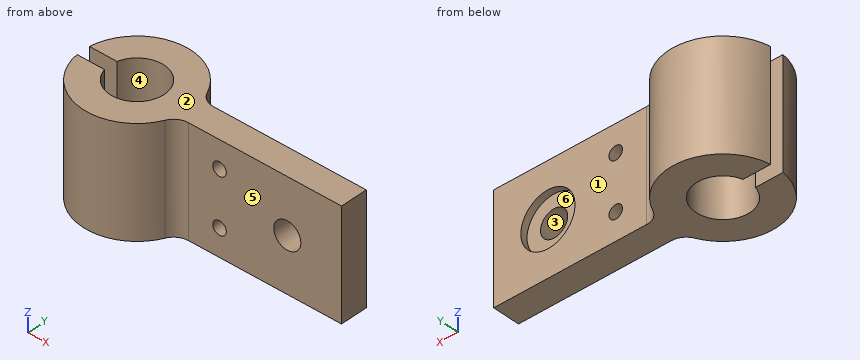
Autodesk Inventor part; units mm, degrees
ref_plane "YZ Plane" through (0, 0, 0) normal (1, 0, 0) x (0, 1, 0)
ref_plane "XZ Plane" through (0, 0, 0) normal (0, 1, 0) x (-1, 0, 0)
ref_plane "XY Plane" through (0, 0, 0) normal (0, 0, 1) x (1, 0, 0)
sketch "Sketch1" plane through (0, 0, 0) normal (0, 0, 1) x (1, 0, 0)
  line L0 (4.5192, 0) -> (76.2, 0)
  line L1 (76.2, 0) -> (76.2, 12.7)
  line L2 (76.2, 12.7) -> (4.5192, 12.7)
  arc A0 (-37.6967, 3.175) -> (-37.6967, 9.525) centre (-25.4, 6.35) ccw
  arc A1 (-2.3852, 17.0962) -> (4.5192, 12.7) centre (4.5192, 20.32) ccw
  arc A2 (4.5192, 0) -> (-2.3852, -4.3962) centre (4.5192, -7.62) ccw
  line L3 (-50.6008, 9.525) -> (-38.1, 9.525)
  line L4 (-50.6008, 3.175) -> (-38.1, 3.175)
  line L5 (-38.1, 9.525) -> (-37.6967, 9.525)
  line L6 (-37.6967, 3.175) -> (-38.1, 3.175)
  arc A3 (-2.3852, 17.0962) -> (-50.6008, 9.525) centre (-25.4, 6.35) ccw
  arc A4 (-50.6008, 3.175) -> (-2.3852, -4.3962) centre (-25.4, 6.35) ccw
  point P0 (0, 0)
  dimension "d0" = 12.7
  dimension "d3" = 25.4
  dimension "d4" = 101.6
  dimension "d5" = 7.62
  dimension "d10" = 25.4
extrude "Extrusion1" add sketch "Sketch1" along normal blind 50.8
sketch "Sketch2" plane through (4.5192, 12.7, 0) normal (0, 1, 0) x (1, 0, 0)
  circle A0 centre (46.2808, -25.4) radius 6.35
  circle A1 centre (14.5308, -12.7) radius 3.175
  circle A2 centre (14.5308, -38.1) radius 3.175
  line L0 (71.6808, 0) -> (71.6808, -50.8)
  line L1 (0, 0) -> (71.6808, 0)
  line L2 (71.6808, -50.8) -> (0, -50.8)
  point P0 (-4.5192, 0)
  dimension "d13" = 12.7
  dimension "d14" = 6.35
  dimension "d15" = 6.35
  dimension "d16" = 25.4
  dimension "d17" = 25.4
  dimension "d18" = 57.15
  dimension "d19" = 12.7
  dimension "d20" = 25.4
  dimension "d21" = 0
extrude "Extrusion2" cut sketch "Sketch2" against normal through all
sketch "Sketch3" plane through (4.5192, 12.7, 0) normal (0, 1, 0) x (1, 0, 0)
  circle A0 centre (46.2808, -25.4) radius 6.35
  circle A1 centre (46.2808, -25.4) radius 12.7
  point P0 (-4.5192, 0)
  dimension "d24" = 25.4
extrude "Extrusion3" cut sketch "Sketch3" against normal blind 3.175
equation "\"d3\" = 2 * d0"
equation "\"d4\" = 8 * d0"
equation "\"d14\" = 0.5 * d13"
equation "\"d15\" = d14"
equation "\"d16\" = d17"
equation "\"d18\" = 2.25 * d16"
equation "\"d19\" = 0.5 * d17"
properties part number "HW 5 Part 4"
Could you check a few things on this model? Use its own coordinates, in mm. Face numbers are marked on the shaded views. A direction names the side the tool comes from. Round coordinates to 2 decimals unless told otherwise and drop trailing zeros. Loops run counter-clockwise (first coordinate to the right, second up) from the corner with the lowest first, then second, coordinate; pieces in that order, holes last. Notation, with made-up numbers: (69, -39.75) - (97, -39.75) arc R15 cw to (97, -17.75) - close; hole circle Ø9 at (-4, -3.5). An arc over 180 degrees is marked (long way). Answer as CSV lines item,"result".
1. Please list where these lines run through material, in increasing order: line 1 along Z through (x, y) = (19, 5); line 2 along Z through (x, y) = (50, 10); line 3 along Y through (x, z) = (-25.4, 39.5). Write a range as [from, to].
Filled in:
line 1,"z = [0, 9.53], [15.87, 34.93], [41.27, 50.8]"
line 2,"z = [0, 12.73], [38.07, 50.8]"
line 3,"y = [-19.05, -6.35], [19.05, 31.75]"
2. I want a section at D-D on y = 6.35. List the corners of the cut face in (x, z) for me (3 decimals), then the cut area to 3 significant figures.
Filled in:
outline,"(-12.7, 0) - (76.2, 0) - (76.2, 50.8) - (-12.7, 50.8) - close; hole circle Ø6.35 at (19.05, 12.7); hole circle Ø6.35 at (19.05, 38.1); hole circle Ø12.7 at (50.8, 25.4)"
area,"4,330 mm^2"
3. I want a section at C-C on x = 50.8. List the corners of the cut face in (y, z) for me (3 decimals).
Filled in:
outline,"(0, 0) - (12.7, 0) - (12.7, 12.7) - (9.525, 12.7) - (9.525, 19.05) - (0, 19.05) - close; (0, 31.75) - (9.525, 31.75) - (9.525, 38.1) - (12.7, 38.1) - (12.7, 50.8) - (0, 50.8) - close"
4. For pin 1 Ø20.5 at (x, z) = (52.5, 19.5) entering from +Y; pin 2 Ø4 at (x, z) = (-47, 19.5) entering from +Y; pin 3 Ø10 at (x, z) = (19.05, 38.1) entering from -Y; pin 4 Ø8 at (x, y) = (14, -3) entering from -Z, each with a flat end and sliding along its axis, tell me the tip position at first contact or that it passes through.
Filled in:
pin 1,"stops at y = 12.7"
pin 2,"stops at y = 22.51"
pin 3,"stops at y = 0"
pin 4,"stops at z = 0"
5. We'd pull the mould along Z, two halves only. Please class the marked faces 1, 2 and 3: +Z half, -Z half, draft (parallel to the pull), parting line (faces both ways), or undercut.
Filled in:
face 1,"draft"
face 2,"+Z half"
face 3,"undercut"
6. I want a section at B-B on z = 25.4. List the corners of the cut face in (x, y) for me (3 decimals), then the cut area to 3 significant figures.
Filled in:
outline,"(-50.601, 3.175) arc R25.4 ccw to (-2.385, -4.396) arc R7.62 cw to (4.519, 0) - (44.45, 0) - (44.45, 9.525) - (38.1, 9.525) - (38.1, 12.7) - (4.519, 12.7) arc R7.62 cw to (-2.385, 17.096) arc R25.4 ccw to (-50.601, 9.525) - (-37.697, 9.525) arc R12.7 cw (long way) to (-37.697, 3.175) - close; (57.15, 0) - (76.2, 0) - (76.2, 12.7) - (63.5, 12.7) - (63.5, 9.525) - (57.15, 9.525) - close"
area,"2,220 mm^2"
7. On a 3-axis mill with a long thin cutter (end or side, diameter ignored), from which of +Z, -Z, +X, -X, +Y, -Y can I reach the whole of each face in a straight line? I mean the marked faces 4, 5 and 6. Say none if no direction works.
Filled in:
face 4,"+Z, -Z"
face 5,"+Z, -Z, +X, -Y"
face 6,"+Y"
8. I want a section at A-A on x = 19.05. List the corners of the cut face in (y, z) for me (3 decimals).
Filled in:
outline,"(0, 0) - (12.7, 0) - (12.7, 9.525) - (0, 9.525) - close; (0, 15.875) - (12.7, 15.875) - (12.7, 34.925) - (0, 34.925) - close; (0, 41.275) - (12.7, 41.275) - (12.7, 50.8) - (0, 50.8) - close"
